Could you check a few things on this model? Use its own coordinates, in mm. Face numbers are marked on the shaded views. A direction names the side the tool comes from. Give positions to 0.01 mm unless a question says otherwise; leave off trailing zeros. Write each loop counter-clockwise with the first axis right and the second up, starting at its lowest first coordinate (ties: lowest second). Pieces come first, ordered by that corner, then holes. Notation, with made-up numbers: M -16,68.25 L -11,68.25 A10 ccw -11,77.25 Z; hole C 77.5,55 d1. An arc over 180 degrees is marked long. Answer as a JSON object with one key per item and string values. Group by question number.
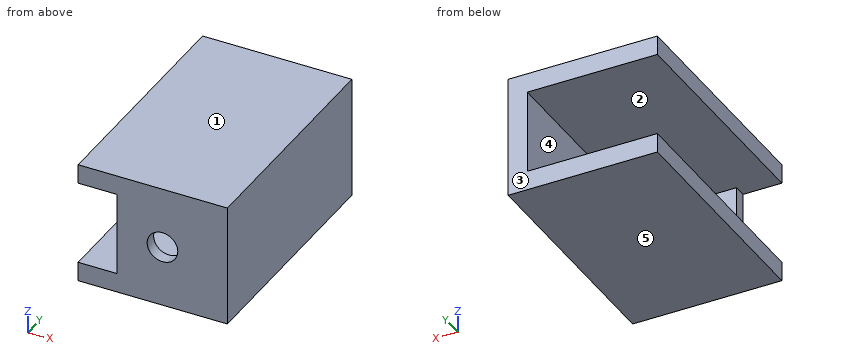
```python
from build123d import *

# Parameters (mm, degrees)
SKETCH2_W               = 16
SKETCH2_H               = 30.7
BOSS_EXTRUDE1_DEPTH     = 9.75
SKETCH3_W               = 10.92
SKETCH3_H               = 29.1
CUT_EXTRUDE1_DEPTH      = 17
SKETCH4_W               = 10.92
SKETCH4_H               = 1.6
CUT_EXTRUDE2_DEPTH      = 5.08
SKETCH5_R               = 2
HOLE_FOR_ACTUATOR_DEPTH = 1.6


with BuildPart() as part:
    # Sketch2 → Boss-Extrude1 (new body, symmetric)
    with BuildSketch(Plane(origin=(0, 0, 0), x_dir=(0, 0, -1), z_dir=(1, 0, 0))):
        Rectangle(SKETCH2_W, SKETCH2_H)
    extrude(amount=BOSS_EXTRUDE1_DEPTH, both=True)

    # Sketch3 → Cut-Extrude1 (cut)
    with BuildSketch(Plane.ZY.offset(9.75)):
        with Locations((0, 0.8)):
            Rectangle(SKETCH3_W, SKETCH3_H)
    extrude(amount=-CUT_EXTRUDE1_DEPTH, mode=Mode.SUBTRACT)

    # Sketch4 → Cut-Extrude2 (cut)
    with BuildSketch(Plane.ZY.offset(9.75)):
        with Locations((0, -14.55)):
            Rectangle(SKETCH4_W, SKETCH4_H)
    extrude(amount=-CUT_EXTRUDE2_DEPTH, mode=Mode.SUBTRACT)

    # Sketch5 → Hole for Actuator (cut)
    with BuildSketch(Plane.XZ.offset(15.35)):
        with Locations((1.27, 0)):
            Circle(SKETCH5_R)
    extrude(amount=-HOLE_FOR_ACTUATOR_DEPTH, mode=Mode.SUBTRACT)


solid = part.part
```
1) Please list where these lines run through material, in increasing order: line 1 along Z through (x, y) = (1.27, -14.75); line 2 along Z through (x, y) = (0.25, 1); line 3 along X through (y, z) = (4, -2.5). Write a range as from..to.
2) If we section it at D-D, the plane y = 8.5: List the corners of the cut face in (x, z) for me.
3) For the marked faces 4 and 5, which set-ups out of +Z, -Z, +X, -X, +Y, -Y let a thin tool reach every point of the face, with its end or its side?
4) If we section it at A-A, the plane z = 0: List the corners of the cut face in (x, y) for me, plus the area to 3 significant figures.
5) If we section it at B-B, the plane x = 1.27: List the corners of the cut face in (y, z) for me.
6) We'd pull the mould along Z, two halves only. Please class the marked faces 1, 2 and 3: released by +Z, released by -Z, zero draft, split by the parting line, or undercut.
7) I'm going to push flat-ended pins straight in: pin 1 (3.5 mm diameter, centred on y = 4.5, z = -2, fed in from -X); pin 2 (1.3 mm diameter, centred on y = -14.5, z = -1.5, fed in from -X); pin 3 (5.5 mm diameter, centred on x = 0.5, z = -2.5, fed in from +Y); pin 4 (3 mm diameter, centred on x = 1.27, z = 0, fed in from +Y). Where does each tip first touch, or does it pass through?
8) If we section it at C-C, the plane z = 4: List the corners of the cut face in (x, y) for me, plus the area to 3 significant figures.
Taken from the geometry:
{
 "1": {"line 1": "-8..-2, 2..8", "line 2": "-8..-5.46, 5.46..8", "line 3": "7.25..9.75"},
 "2": {"outline": "M -9.75,-8 L 9.75,-8 L 9.75,8 L -9.75,8 L -9.75,5.46 L 7.25,5.46 L 7.25,-5.46 L -9.75,-5.46 Z"},
 "3": {"face 4": "-X, +Y", "face 5": "-Z, +X, -X, +Y, -Y"},
 "4": {"outline": "M -4.67,-15.35 L -0.73,-15.35 L -0.73,-13.75 L -4.67,-13.75 Z; M 3.27,-15.35 L 9.75,-15.35 L 9.75,15.35 L 7.25,15.35 L 7.25,-13.75 L 3.27,-13.75 Z", "area": "89.4 mm²"},
 "5": {"outline": "M -15.35,-8 L 15.35,-8 L 15.35,-5.46 L -13.75,-5.46 L -13.75,-2 L -15.35,-2 Z; M -15.35,2 L -13.75,2 L -13.75,5.46 L 15.35,5.46 L 15.35,8 L -15.35,8 Z"},
 "6": {"face 1": "released by +Z", "face 2": "undercut", "face 3": "zero draft"},
 "7": {"pin 1": "x = 7.25", "pin 2": "x = -4.67", "pin 3": "y = -13.75", "pin 4": "through"},
 "8": {"outline": "M -4.67,-15.35 L 9.75,-15.35 L 9.75,15.35 L 7.25,15.35 L 7.25,-13.75 L -4.67,-13.75 Z", "area": "95.8 mm²"}
}
